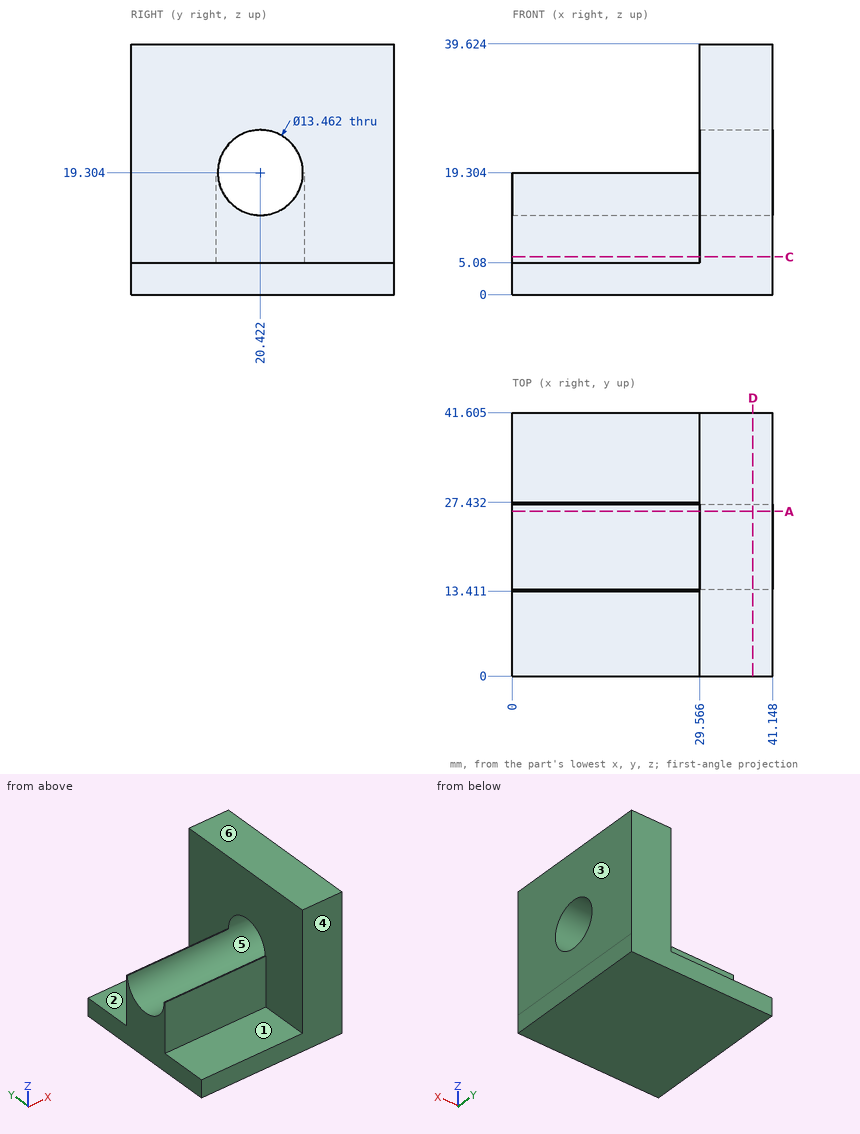
Could you check a few things on this drawing? It's one solid part, dimensions in mm from its lowest x, y, z. A direction names the side the tool comes from. Coordinates: 2 decimals unless noted, no trailing zeros. Order: outer loops, then holes, each group sorted by start corner. A loop starts at its lowest first (then second) coordinate and runs counter-clockwise, first axis right, second up. Notation, with made-up numbers: (-28.75, 42) - (-15.75, 42) arc R27 cw to (-15.75, 73) - close; hole circle Ø9 at (49, 62). An arc over 180 degrees is marked (long way). One line per question, with ' | ' between items.
(1) Suppose I cut it at C-C on z = 6. List the corners of the cut face in (x, y) for me (1 decimal).
Report:
outline: (0, 13.4) - (29.6, 13.4) - (29.6, 0) - (41.1, 0) - (41.1, 41.6) - (29.6, 41.6) - (29.6, 27.4) - (0, 27.4) - close
(2) Will these pins go through, and if not, where does the flat tip stop? pin 1 (7 mm diameter, centred on x = 12, z = 15, fed in from -Y); pin 2 (15.5 mm diameter, centred on x = 14, y = 36.5, fed in from +Z); pin 3 (4.5 mm diameter, centred on x = 16.5, z = 14, fed in from +Y).
Report:
pin 1: stops at y = 13.41 | pin 2: stops at z = 5.08 | pin 3: stops at y = 27.43
(3) For the marked faces 1, 2 and 3, which set-ups out of +Z, -Z, +X, -X, +Y, -Y let a thin tool reach every point of the face, with its end or its side?
Report:
face 1: +Z, -X, -Y | face 2: +Z, -X, +Y | face 3: +Z, -Z, +X, +Y, -Y
(4) If we mould it in two halves opening along Y, with no side actions, what happens to the marked faces 4, 5 and 6? For each: pulls with the +Y half, pulls with the -Y half, needs draft (parallel to the pull), parting line crosses it, or undercut.
Report:
face 4: pulls with the -Y half | face 5: undercut | face 6: needs draft
(5) If I drill on L1, parallel to Z at x = 3, y = 2; L2, parallel to X at y = 29, z = 14.5 (1 decimal); L3, parallel to Y at x = 24, z = 7.5, over which ranges is the centre line in solid material (lowest first)?
Report:
L1: z = 0 to 5.08 | L2: x = 29.6 to 41.1 | L3: y = 13.41 to 27.43
(6) Suppose I cut it at D-D on x = 38. List the corners of the cut face in (y, z) for me (1 decimal), and give its area (3 significant figures).
Report:
outline: (0, 0) - (41.6, 0) - (41.6, 39.6) - (0, 39.6) - close; hole circle Ø13.5 at (20.4, 19.3) | area: 1,510 mm2
(7) Suppose I cut it at A-A on y = 26. List the corners of the cut face in (x, z) for me (1 decimal).
Report:
outline: (0, 0) - (41.1, 0) - (41.1, 15.5) - (0, 15.5) - close; (29.6, 23.1) - (41.1, 23.1) - (41.1, 39.6) - (29.6, 39.6) - close
